Geometry: final body of the model. Coordinates: model frame, mm. Face numbers are marked on the shaded views. A direction names the side the tool comes from. Round coordinates to 2 decimals unless told otherwise and drop trailing zeros. Loops run counter-clockwise (first coordinate to the right, second up) from the corner with the lowest first, then second, coordinate; pieces in that order, holes last. Notation, with made-up numbers: M 63.5,74 L 86.5,74 A17 cw 86.5,99 Z; hole C 47.5,19 d2. An arc over 180 degrees is marked long. Return JSON: item names as keys, results as strings.
from build123d import *

# Parameters (mm, degrees)
F0_W     = 43
F0_H     = 33
F0_W_2   = 39
F0_H_2   = 29
F1_DEPTH = 15
F0_R     = 1.1
F2_DEPTH = 2
F3_DEPTH = 7
F4_R     = 4
F5_DEPTH = 2
F6_W     = 29
F6_H     = 11
F7_DEPTH = 2
F8_W     = 27.5
F8_H     = 24.9
F9_DEPTH = 5
F11_D    = 2.4
F13_D    = 2.4


with BuildPart() as f1:
    # F0 (on Top) → F1 (new body)
    with BuildSketch(Plane.XY):
        Rectangle(F0_W, F0_H)
        Rectangle(F0_W_2, F0_H_2, mode=Mode.SUBTRACT)
    extrude(amount=F1_DEPTH)

    # F0 (on Top) → F2 (join)
    with BuildSketch(Plane.XY):
        Rectangle(F0_W_2, F0_H_2)
        with Locations((15.5, -10.16)):
            Circle(F0_R, mode=Mode.SUBTRACT)
        with Locations((15.5, 10.16)):
            Circle(F0_R, mode=Mode.SUBTRACT)
    extrude(amount=F2_DEPTH)

    # F0 (on Top) → F3 (join)
    with BuildSketch(Plane.XY):
        with Locations((15.5, -10.16)):
            Circle(F0_R)
        with Locations((15.5, 10.16)):
            Circle(F0_R)
    extrude(amount=F3_DEPTH)

    # F4 (on face) → F5 (cut, through all)
    with BuildSketch(Plane.YZ.offset(21.5)):
        with Locations((0, 7.5)):
            Circle(F4_R)
    extrude(amount=-F5_DEPTH, mode=Mode.SUBTRACT)

    # F6 (on face) → F7 (cut, through all)
    with BuildSketch(Plane(origin=(-21.5, 0, 0), x_dir=(0, -1, 0), z_dir=(-1, 0, 0))):
        with Locations((0, 7.5)):
            Rectangle(F6_W, F6_H)
    extrude(amount=-F7_DEPTH, mode=Mode.SUBTRACT)

    # F8 (on face) → F9 (join)
    with BuildSketch(Plane(origin=(0, 0, 0), x_dir=(1, 0, 0), z_dir=(0, 0, -1))):
        with Locations((5.75, 0)):
            Rectangle(F8_W, F8_H)
        with BuildLine():
            Line((6.75, 9.45), (16.5, 9.45))
            Line((16.5, 9.45), (16.5, 1))
            ThreePointArc((16.5, 1), (17.2071067812, 0.7071067812), (17.5, 0))
            ThreePointArc((17.5, 0), (17.2071067812, -0.7071067812), (16.5, -1))
            Line((16.5, -1), (16.5, -9.45))
            Line((16.5, -9.45), (6.75, -9.45))
            ThreePointArc((6.75, -9.45), (5.75, -10.45), (4.75, -9.45))
            Line((4.75, -9.45), (-5, -9.45))
            Line((-5, -9.45), (-5, -1))
            ThreePointArc((-5, -1), (-6, 0), (-5, 1))
            Line((-5, 1), (-5, 9.45))
            Line((-5, 9.45), (4.75, 9.45))
            ThreePointArc((4.75, 9.45), (5.75, 10.45), (6.75, 9.45))
        make_face(mode=Mode.SUBTRACT)
        with BuildLine():
            ThreePointArc((17.5, 0), (17.2071067812, 0.7071067812), (16.5, 1))
            Line((16.5, 1), (16.5, -1))
            ThreePointArc((16.5, -1), (17.2071067812, -0.7071067812), (17.5, 0))
        make_face()
        with BuildLine():
            Line((16.5, -1), (16.5, 1))
            ThreePointArc((16.5, 1), (15.5, 0), (16.5, -1))
        make_face()
        with BuildLine():
            Line((4.75, -9.45), (6.75, -9.45))
            ThreePointArc((6.75, -9.45), (5.75, -8.45), (4.75, -9.45))
        make_face()
        with BuildLine():
            ThreePointArc((4.75, -9.45), (5.75, -10.45), (6.75, -9.45))
            Line((6.75, -9.45), (4.75, -9.45))
        make_face()
        with BuildLine():
            ThreePointArc((4.75, 9.45), (5.75, 8.45), (6.75, 9.45))
            Line((6.75, 9.45), (4.75, 9.45))
        make_face()
        with BuildLine():
            Line((4.75, 9.45), (6.75, 9.45))
            ThreePointArc((6.75, 9.45), (5.75, 10.45), (4.75, 9.45))
        make_face()
        with BuildLine():
            ThreePointArc((-4, 0), (-4.2928932188, 0.7071067812), (-5, 1))
            Line((-5, 1), (-5, -1))
            ThreePointArc((-5, -1), (-4.2928932188, -0.7071067812), (-4, 0))
        make_face()
        with BuildLine():
            Line((-5, -1), (-5, 1))
            ThreePointArc((-5, 1), (-6, 0), (-5, -1))
        make_face()
    extrude(amount=F9_DEPTH)

    # F11 (through all)
    with Locations(Plane.YZ.offset(19.5)):
        with Locations((0, -2.5)):
            Hole(F11_D / 2)

    # F13 (through all)
    with Locations(Plane(origin=(0, 12.45, 0), x_dir=(-1, 0, 0), z_dir=(0, 1, 0))):
        with Locations((-5.75, -2.5)):
            Hole(F13_D / 2)


solid = f1.part
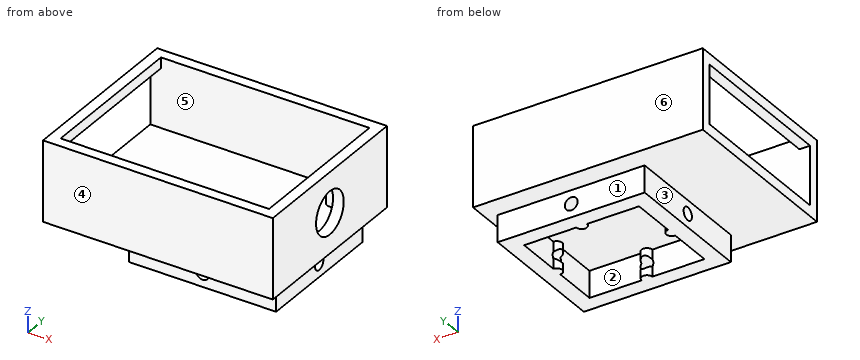
Q1. Material intervals for L1, parallel to Y at x = 4, z = 8.5; L2, parallel to Y at x = 16.95, z = -2.5; L3, parallel to Z at x = 17, y = 0, sorted ascending.
Determined:
{"L1": "y = -16.5 to -14.5, 14.5 to 16.5", "L2": "y = -12.45 to -1.2, 1.2 to 12.45", "L3": "z = -5 to -3.7, -1.3 to 2"}
Q2. Pin query (flat end, axial travel): pin 1 (1.9 mm diameter, centred on y = 0, z = -2.5, fed in from +X); pin 2 (1.5 mm diameter, centred on y = 4, z = -3.5, fed in from +X); pin 3 (2.5 mm diameter, centred on x = 10, z = -2.5, fed in from +Y); pin 4 (2.5 mm diameter, centred on x = 16, y = -10.5, fed in from +Z). Return the tip coordinate at first contact, or that it passes through.
Determined:
{"pin 1": "passes through", "pin 2": "stops at x = 19.5", "pin 3": "stops at y = 12.45", "pin 4": "stops at z = 7"}
Q3. Section query A-A (z = 7.5). Output: boundary loops of the cut face in (x, y).
Determined:
{"outline": "M -21.5,-16.5 L 21.5,-16.5 L 21.5,-4 L 19.5,-4 L 19.5,-14.5 L -21.5,-14.5 Z; M -21.5,14.5 L 19.5,14.5 L 19.5,4 L 21.5,4 L 21.5,16.5 L -21.5,16.5 Z"}
Q4. Reachability of the marked faces 1, 2 and 3 from +Z, -Z, +X, -X, +Y, -Y: full face, straight path, thin tool, end or side. Return the list, or none.
Determined:
{"face 1": "-Z, +X, -X, +Y", "face 2": "-Z", "face 3": "-Z, -X, +Y, -Y"}
Q5. Section query D-D (x = 19). Output: boundary loops of the cut face in (y, z).
Determined:
{"outline": "M -16.5,0 L -12.45,0 L -12.45,-5 L 12.45,-5 L 12.45,0 L 16.5,0 L 16.5,15 L 14.5,15 L 14.5,2 L -14.5,2 L -14.5,15 L -16.5,15 Z; hole C 0,-2.5 d2.4"}
Q6. Pull-direction query (Y, two-part tool) for the marked faces 4, 5 and 6; classes: pulls with the +Y half, pulls with the -Y half, needs draft (parallel to the pull), parting line crosses it, or undercut.
Determined:
{"face 4": "pulls with the -Y half", "face 5": "undercut", "face 6": "pulls with the +Y half"}
Q7. Section query B-B (y = 10.16). Output: boundary loops of the cut face in (x, z).
Determined:
{"outline": "M -21.5,0 L -8,0 L -8,-5 L 19.5,-5 L 19.5,0 L 21.5,0 L 21.5,15 L 19.5,15 L 19.5,2 L 16.6,2 L 16.6,7 L 14.4,7 L 14.4,2 L -21.5,2 Z; M -21.5,13 L -19.5,13 L -19.5,15 L -21.5,15 Z; hole C 5.75,-2.5 d2.4"}
Q8. Section query C-C (x = 5.75). Output: boundary loops of the cut face in (y, z).
Determined:
{"outline": "M -16.5,0 L -12.45,0 L -12.45,-1.3 L -8.45,-1.3 L -8.45,0 L 8.45,0 L 8.45,-1.3 L 12.45,-1.3 L 12.45,0 L 16.5,0 L 16.5,15 L 14.5,15 L 14.5,2 L -14.5,2 L -14.5,15 L -16.5,15 Z; M -12.45,-5 L -8.45,-5 L -8.45,-3.7 L -12.45,-3.7 Z; M 8.45,-5 L 12.45,-5 L 12.45,-3.7 L 8.45,-3.7 Z"}
